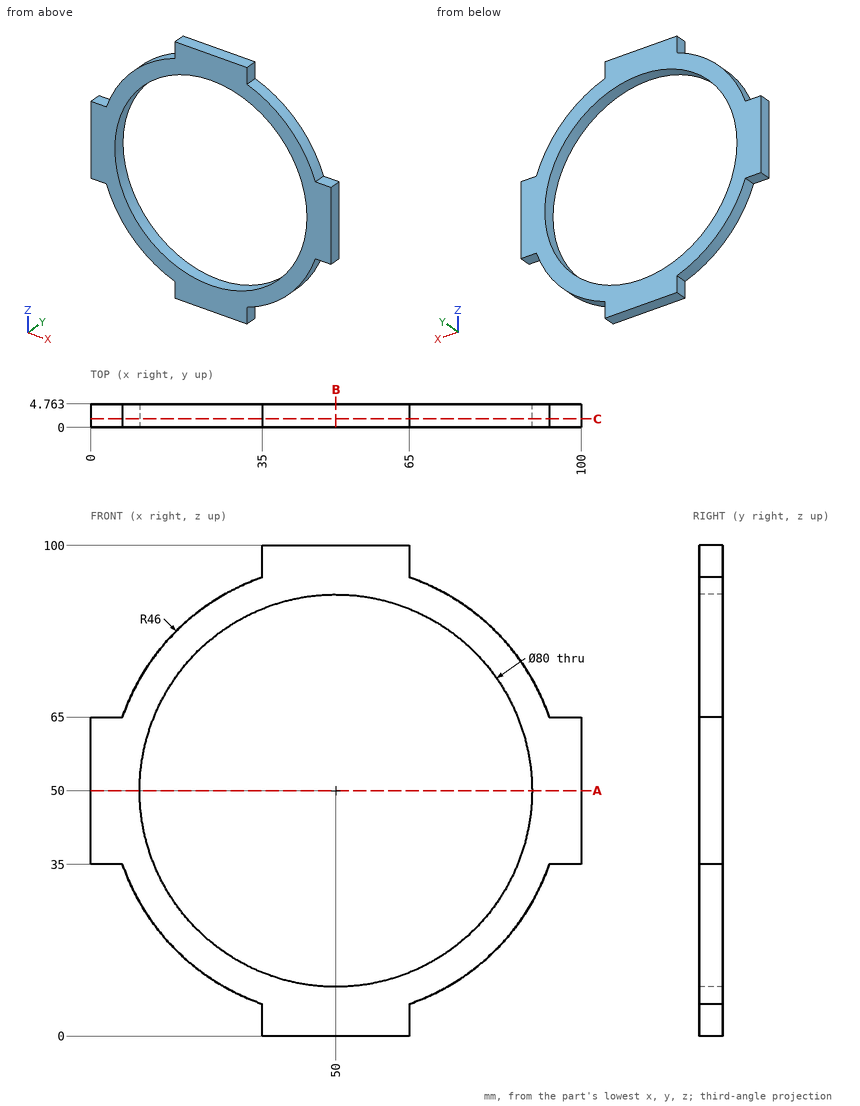
Job drawing, mm, ordinate dimensions from the low corner. One solid piece. Round coordinates to 2 decimals unless told otherwise and drop trailing zeros. Loops run counter-clockwise (first coordinate to the right, second up) from the corner with the lowest first, then second, coordinate; pieces in that order, holes last.
Item 1: Cut at A-A, the plane z = 50. Give the cut face in (x, y).
Item 2: Cut at B-B, the plane x = 50. Give the cut face in (y, z).
Item 3: Cut at C-C, the plane y = 1.75. Give the cut face in (x, z) (1 decimal).
Item 4: Drill centre lines: line 1 (Z direction, x = 50, y = 2.5); line 2 (X direction, y = 2.15, z = 51); line 3 (Z direction, x = 58, y = 3.15). Where is each one in solid material? Low to high.
Item 5: Drop flat-ended pins along their axis: P1, Ø1.4, axis at y = 1.5, z = 4, coming from the +X side; P2, Ø2, axis at y = 3, z = 17.5, coming from the -X side; P3, Ø1.4, axis at x = 3.5, y = 3, coming from the -Z side. Give the stop position or say it passes through.
A:
1. outline: (0, 0) - (10, 0) - (10, 4.76) - (0, 4.76) - close; (90, 0) - (100, 0) - (100, 4.76) - (90, 4.76) - close
2. outline: (0, 0) - (4.76, 0) - (4.76, 10) - (0, 10) - close; (0, 90) - (4.76, 90) - (4.76, 100) - (0, 100) - close
3. outline: (0, 35) - (6.5, 35) arc R46 ccw to (35, 6.5) - (35, 0) - (65, 0) - (65, 6.5) arc R46 ccw to (93.5, 35) - (100, 35) - (100, 65) - (93.5, 65) arc R46 ccw to (65, 93.5) - (65, 100) - (35, 100) - (35, 93.5) arc R46 ccw to (6.5, 65) - (0, 65) - close; hole circle Ø80 at (50, 50)
4. line 1: z = 0 to 10, 90 to 100
4. line 2: x = 0 to 10.01, 89.99 to 100
4. line 3: z = 0 to 10.81, 89.19 to 100
5. P1: stops at x = 65
5. P2: stops at x = 16.48
5. P3: stops at z = 35
